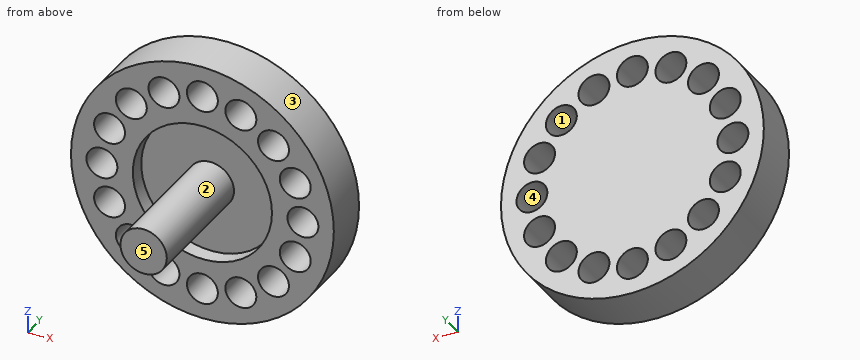
from build123d import *

# Parameters (mm, degrees)
F0_R     = 8.5
F0_R_2   = 4.5
F1_DEPTH = 3
F2_R     = 1
F3_DEPTH = 5
F4_R     = 4.5
F5_DEPTH = 2
F6_R     = 1.5
F7_DEPTH = 8


with BuildPart() as f1:
    # F0 (on Front) → F1 (new body)
    with BuildSketch(Plane.XZ):
        Circle(F0_R)
        Circle(F0_R_2, mode=Mode.SUBTRACT)
    extrude(amount=F1_DEPTH)

    # F2 (on face) → F3 (cut)
    with BuildSketch(Plane.XZ.offset(3)):
        with Locations((0, 6.5)):
            Circle(F2_R)
        with Locations((2.487442, 6.005217)):
            Circle(F2_R)
        with Locations((4.596194, 4.596194)):
            Circle(F2_R)
        with Locations((6.005217, 2.487442)):
            Circle(F2_R)
        with Locations((6.5, 0)):
            Circle(F2_R)
        with Locations((6.005217, -2.487442)):
            Circle(F2_R)
        with Locations((4.596194, -4.596194)):
            Circle(F2_R)
        with Locations((2.487442, -6.005217)):
            Circle(F2_R)
        with Locations((0, -6.5)):
            Circle(F2_R)
        with Locations((-2.487442, -6.005217)):
            Circle(F2_R)
        with Locations((-4.596194, -4.596194)):
            Circle(F2_R)
        with Locations((-6.005217, -2.487442)):
            Circle(F2_R)
        with Locations((-6.5, 0)):
            Circle(F2_R)
        with Locations((-6.005217, 2.487442)):
            Circle(F2_R)
        with Locations((-4.596194, 4.596194)):
            Circle(F2_R)
        with Locations((-2.487442, 6.005217)):
            Circle(F2_R)
    extrude(amount=-F3_DEPTH, mode=Mode.SUBTRACT)

    # F4 (on Front) → F5 (join)
    with BuildSketch(Plane.XZ):
        Circle(F4_R)
    extrude(amount=F5_DEPTH)

    # F6 (on face) → F7 (join)
    with BuildSketch(Plane.XZ.offset(2)):
        Circle(F6_R)
    extrude(amount=F7_DEPTH)


solid = f1.part
Input: part model. Units: mm. Frame: model coordinates. Face numbers are marked on the shaded views. A direction names the side the tool comes from. Give positions to 0.01 mm unless a question says otherwise; leave off trailing zeros. Write each loop counter-clockwise with the first axis right and the second up, starting at its lowest first coordinate (ties: lowest second). Pieces come first, ordered by that corner, then holes.
Q1. Pull-direction query (X, two-part tool) for the marked faces 3, 4 and 5; classes: pulls with the +X half, pulls with the -X half, needs draft (parallel to the pull), parting line crosses it, or undercut.
Q2. Material intervals for probe 1 along Z at (x, y) = (0, -2.5); probe 2 along Z at (x, y) = (0, -0.7); probe 3 along X at (y, z) = (-2, 6.75), sorted ascending.
Q3. Section B-B, the plane z = 4. Output: boundary loops of the cut face in (x, y), plus the area to 3 significant figures.
Q4. First-contact query: P1, Ø1.5, axis at x = 1.5, y = -5, coming from the -Z side; P2, Ø3, axis at x = 4.6, z = -4.6, coming from the -Y side; P3, Ø3, axis at y = -3, z = 5, coming from the +X side. Flat tips, straight axial feed; report the tip coordinate or a pass-through.
Q5. Set-up query: the marked faces 1 and 2. Return all of +Z, -Z, +X, -X, +Y, -Y with unobstructed straight access to the full face (end or side cutting, diameter ignored); none if empty.
Q6. Section D-D, the plane z = 6.5. Output: boundary loops of the cut face in (x, y), plus the area to 3 significant figures.
Q7. Section A-A, the plane x = 0. Output: boundary loops of the cut face in (y, z), plus the area to 3 significant figures.
Q8. Section C-C, the plane x = 6.25. Output: boundary loops of the cut face in (y, z).
Filled in:
1. face 3: parting line crosses it
1. face 4: undercut
1. face 5: needs draft
2. probe 1: z = -8.5 to -7.5, -5.5 to -4.5, -1.5 to 1.5, 4.5 to 5.5, 7.5 to 8.5
2. probe 2: z = -8.5 to -7.5, -5.5 to 5.5, 7.5 to 8.5
2. probe 3: x = -5.17 to -3.15, -1.82 to -0.97, 0.97 to 1.82, 3.15 to 5.17
3. outline: (-7.5, -3) - (-5.4, -3) - (-5.4, 0) - (-7.5, 0) - close; (-3.79, -3) - (-2.06, -3) - (-2.06, -2) - (2.06, -2) - (2.06, -3) - (3.79, -3) - (3.79, 0) - (-3.79, 0) - close; (5.4, -3) - (7.5, -3) - (7.5, 0) - (5.4, 0) - close
3. area: 31.2 mm2
4. P1: stops at z = -1.3
4. P2: stops at y = -3
4. P3: stops at x = 7.75
5. face 1: +Y, -Y
5. face 2: -Y
6. outline: (-5.48, -3) - (-3.36, -3) - (-3.36, 0) - (-5.48, 0) - close; (-1.62, -3) - (-1, -3) - (-1, 0) - (-1.62, 0) - close; (1, -3) - (1.62, -3) - (1.62, 0) - (1, 0) - close; (3.36, -3) - (5.48, -3) - (5.48, 0) - (3.36, 0) - close
6. area: 16.4 mm2
7. outline: (-10, -1.5) - (-2, -1.5) - (-2, -4.5) - (-3, -4.5) - (-3, -5.5) - (0, -5.5) - (0, 5.5) - (-3, 5.5) - (-3, 4.5) - (-2, 4.5) - (-2, 1.5) - (-10, 1.5) - close; (-3, -8.5) - (0, -8.5) - (0, -7.5) - (-3, -7.5) - close; (-3, 7.5) - (0, 7.5) - (0, 8.5) - (-3, 8.5) - close
7. area: 54.0 mm2
8. outline: (-3, -5.76) - (0, -5.76) - (0, -3.46) - (-3, -3.46) - close; (-3, -1.52) - (0, -1.52) - (0, -0.97) - (-3, -0.97) - close; (-3, 0.97) - (0, 0.97) - (0, 1.52) - (-3, 1.52) - close; (-3, 3.46) - (0, 3.46) - (0, 5.76) - (-3, 5.76) - close
